The drawing under review shows one solid part. Ordinate dimensions are in mm from its lowest x, y, z. A direction names the side the tool comes from. Round coordinates to 2 decimals unless told otherwise and drop trailing zeros. Order: outer loops, then holes, each group sorted by start corner. A loop starts at its lowest first (then second) coordinate and runs counter-clockwise, first axis right, second up. Notation, with made-up numbers: M -39,72.25 L -7,72.25 A9 ccw -7,78.25 Z; hole C 62.5,2 d1. An arc over 180 degrees is marked long. Answer as a JSON object with one key per item and string values. Group by question number.
1. Machinability: for the marked faces 1, 2 and 3, which of the approach directions +Z, -Z, +X, -X, +Y, -Y give a long, thin tool a straight path to every point of the face, cutting with its end or side? Answer none if there is none.
2. Add section A-A on y = 15. State the section outline as (x, z) points, and give its area (3 significant figures).
3. Add section C-C on x = 120. State the section outline as (y, z) points.
4. Add section B-B on z = 6.75. State the section outline as (x, y) points.
5. To check wall thickness, follow probe 1 along Y at (x, z) = (120, 8); probe 2 along X at (y, z) = (12, 2.5); probe 3 along Y at (x, z) = (118, 10). State the ranges of each line that lie inside material, in increasing order. Write a range as [from, to].
6. Clearance check with flat-ended pins moving along their axes: P1, Ø4, axis at y = 12, z = 13.5, coming from the +X side; P2, Ø6, axis at x = 23.5, y = 28.5, coming from the +Z side; P3, Ø1.8, axis at y = 31.5, z = 12, coming from the -X side. State where each tip first meets the part, or that it passes through.
7. Add section D-D on y = 48. State the section outline as (x, z) points, and give its area (3 significant figures).
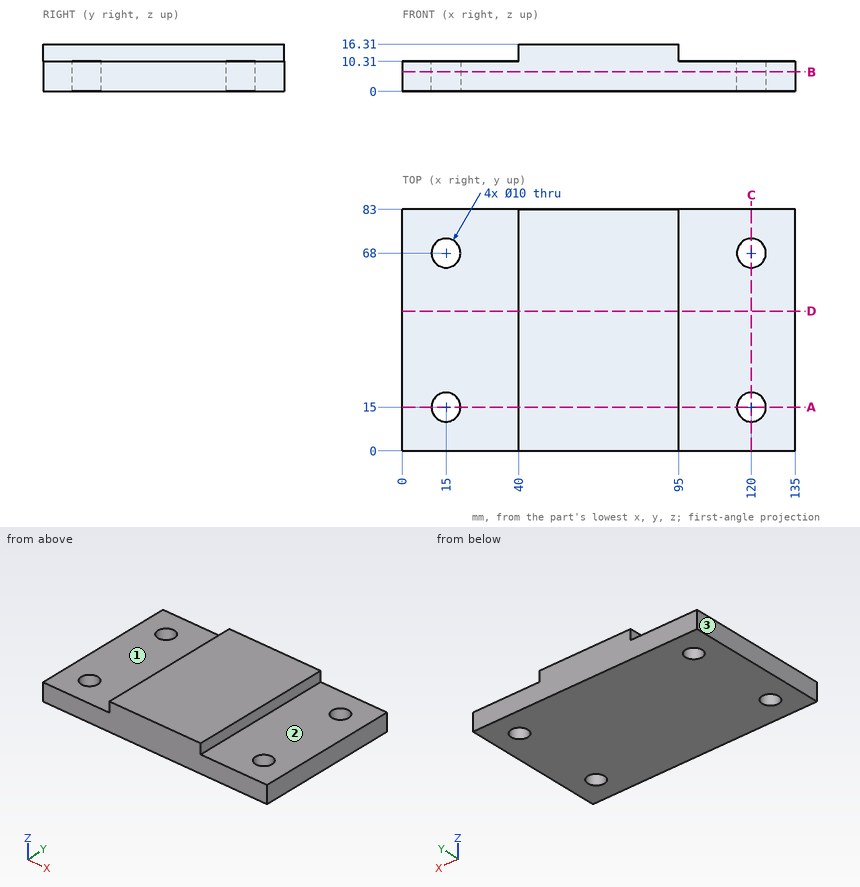
Recorded:
{
 "1": {"face 1": "+Z, -X, +Y, -Y", "face 2": "+Z, +X, +Y, -Y", "face 3": "+Z, -Z, -X, +Y, -Y"},
 "2": {"outline": "M 0,0 L 10,0 L 10,10.31 L 0,10.31 Z; M 20,0 L 115,0 L 115,10.31 L 95,10.31 L 95,16.31 L 40,16.31 L 40,10.31 L 20,10.31 Z; M 125,0 L 135,0 L 135,10.31 L 125,10.31 Z", "area": "1,520 mm²"},
 "3": {"outline": "M 0,0 L 10,0 L 10,10.31 L 0,10.31 Z; M 20,0 L 63,0 L 63,10.31 L 20,10.31 Z; M 73,0 L 83,0 L 83,10.31 L 73,10.31 Z"},
 "4": {"outline": "M 0,0 L 135,0 L 135,83 L 0,83 Z; hole C 15,15 d10; hole C 15,68 d10; hole C 120,15 d10; hole C 120,68 d10"},
 "5": {"probe 1": "y = [0, 10], [20, 63], [73, 83]", "probe 2": "x = [0, 11], [19, 116], [124, 135]", "probe 3": "y = [0, 10.42], [19.58, 63.42], [72.58, 83]"},
 "6": {"P1": "stops at x = 95", "P2": "stops at z = 10.31", "P3": "stops at x = 40"},
 "7": {"outline": "M 0,0 L 135,0 L 135,10.31 L 95,10.31 L 95,16.31 L 40,16.31 L 40,10.31 L 0,10.31 Z", "area": "1,720 mm²"}
}
